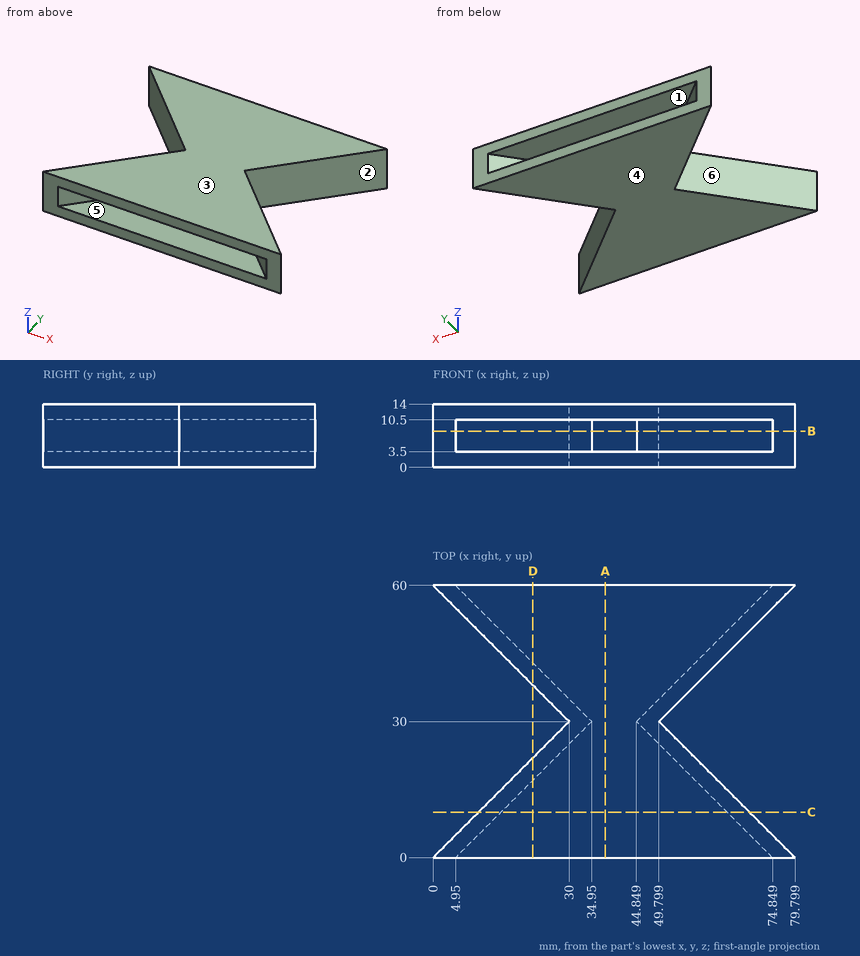
Job drawing, mm, ordinate dimensions from the low corner. One solid piece. A direction names the side the tool comes from. Round coordinates to 2 decimals unless told otherwise and drop trailing zeros. Loops run counter-clockwise (first coordinate to the right, second up) from the corner with the lowest first, then second, coordinate; pieces in that order, holes last.
(1) Cut at D-D (x = 22). Give the cut face in (y, z), plus the area to 3 significant figures.
(2) Which spindle directions (+Z, -Z, +X, -X, +Y, -Y) get a long thin tool onto all of the face, cutting with end or side? Do the marked faces 4, 5 and 6. Say none if no direction does.
(3) Two-plate mould, pull along X, no slides. Class the marked faces 1, 2 and 3: +X half, -X half, draft (parallel to the pull), parting line (faces both ways), or undercut.
(4) Cut at C-C (y = 10). Give the cut face in (x, z), plus the area to 3 significant figures.
(5) Cut at A-A (x = 38). Give the cut face in (y, z), plus the area to 3 significant figures.
(6) Cut at B-B (z = 8). Give the cut face in (x, y).
(7) Drop flat-ended pins along their axis: pin 1 (6 mm diameter, centred on y = 19, z = 11.5, fed in from +X); pin 2 (1.5 mm diameter, centred on y = 29.5, z = 7.5, fed in from +X); pin 3 (3 mm diameter, centred on x = 27, z = 5.5, fed in from +Y). Give the stop position or say it passes through.
(8) Wall check: line 1 along Z through (x, y) = (49.5, 3.5); line 2 along Y through (x, z) = (15.5, 7.5); line 3 along X through (y, z) = (47.5, 5.25). Give the ranges that are in metal, low to high.
Findings below:
1. outline: (0, 0) - (22, 0) - (22, 14) - (0, 14) - (0, 10.5) - (17.05, 10.5) - (17.05, 3.5) - (0, 3.5) - close; (38, 0) - (60, 0) - (60, 3.5) - (42.95, 3.5) - (42.95, 10.5) - (60, 10.5) - (60, 14) - (38, 14) - close
1. area: 377 mm2
2. face 4: -Z, +X, -X, +Y, -Y
2. face 5: none
2. face 6: +Z, -Z, -X
3. face 1: undercut
3. face 2: +X half
3. face 3: draft
4. outline: (10, 0) - (69.8, 0) - (69.8, 14) - (10, 14) - close; hole (14.95, 3.5) - (64.85, 3.5) - (64.85, 10.5) - (14.95, 10.5) - close
4. area: 488 mm2
5. outline: (0, 0) - (60, 0) - (60, 3.5) - (0, 3.5) - close; (0, 10.5) - (60, 10.5) - (60, 14) - (0, 14) - close
5. area: 420 mm2
6. outline: (0, 0) - (4.95, 0) - (34.95, 30) - (4.95, 60) - (0, 60) - (30, 30) - close; (44.85, 30) - (74.85, 0) - (79.8, 0) - (49.8, 30) - (79.8, 60) - (74.85, 60) - close
7. pin 1: stops at x = 63.8
7. pin 2: stops at x = 51.05
7. pin 3: stops at y = 39.45
8. line 1: z = 0 to 3.5, 10.5 to 14
8. line 2: y = 10.55 to 15.5, 44.5 to 49.45
8. line 3: x = 12.5 to 17.45, 62.35 to 67.3
